The listing builds one solid part. Answer for the finished solid, in the listing's coordinates (mm). A direction names the side the tool comes from. Coordinates: 2 decimals unless noted, no trailing zeros. Order: outer loops, then holes, each group sorted by start corner. A loop starts at its lowest first (then second) coordinate and runs counter-clockwise, first axis right, second up. Notation, with made-up numbers: (16, -22) -> (66, -22) arc R24 cw to (66, -1) -> close; hole circle Ø2 at (-39, 12). An arc over 180 degrees is marked (long way). Answer in a Markdown table with one row per item.
```python
from build123d import *

# Parameters (mm, degrees)
CUT_EXTRUDE2_DEPTH      = 28.696934518
CUT_EXTRUDE2_DEPTH_BACK = 28.696934518
SKETCH10_R              = 0.75


with BuildPart() as part:
    # Sketch1 → Revolve1 (revolve)
    with BuildSketch(Plane(origin=(0, 0, 0), x_dir=(0, 0, -1), z_dir=(1, 0, 0))):
        Polygon((-6.059175667, 3.611199877), (-6.059175667, -4.388800123), (-4.559175656, -4.388756431), (-4.559175656, -2.888756431), (-3.059175668, -2.88856746), (-3.059175668, -4.388756431), (-1.059175668, -4.388756431), (-0.059175667, -1.888800123), (-0.059175667, 0.111199877), (-0.809175667, 0.611199877), (-0.809175667, 3.611199877), align=None)
    revolve(axis=Axis((0, 4.111199877, -8.940824333), (0, -1, 0)))

    # Sketch10 → Cut-Extrude2 (cut, two sides: drawn at the far end of the back side and taken through both)
    with BuildSketch(Plane(origin=(0, 5.926037439, -14.814834675), x_dir=(1, 0, 0), z_dir=(0, -0.37139627193644054, 0.9284744526327656)).offset(-CUT_EXTRUDE2_DEPTH_BACK)):
        with Locations(Location((4.041684761, -9.017, 0), (0, 0, 270))):
            Circle(SKETCH10_R)
    extrude(amount=CUT_EXTRUDE2_DEPTH + CUT_EXTRUDE2_DEPTH_BACK, mode=Mode.SUBTRACT)


solid = part.part
```
(1) A cutting plane is placed at A-A, the plane x = 0. Determine the outline of the cut face in (y, z), then the cut area to 3 significant figures.
Check values:
| item | result |
|---|---|
| outline | (-4.39, -23.94) -> (3.61, -23.94) -> (3.61, -18.69) -> (0.61, -18.69) -> (0.11, -17.94) -> (-1.89, -17.94) -> (-4.39, -18.94) -> (-4.39, -20.94) -> (-2.89, -20.94) -> (-2.89, -22.44) -> (-4.39, -22.44) -> close; (-4.39, 1.06) -> (-1.89, 0.06) -> (0.11, 0.06) -> (0.61, 0.81) -> (3.61, 0.81) -> (3.61, 6.06) -> (-4.39, 6.06) -> (-4.39, 4.56) -> (-2.89, 4.56) -> (-2.89, 3.06) -> (-4.39, 3.06) -> close |
| area | 84.1 mm² |
(2) Flat-ended cylindrical pins translate along their axes: pin 1 (15.5 mm diameter, centred on x = 0, z = -8.94, fed in from +Y) (3 decimals); pin 2 (1 mm diameter, centred on x = 3, z = 0.5, fed in from -Y); pin 3 (1 mm diameter, centred on y = 0, z = -15, fed in from +X). Find the tip coordinate at first contact, or state that the pin passes through.
Check values:
| item | result |
|---|---|
| pin 1 | through |
| pin 2 | y = -4.39 |
| pin 3 | x = 13.93 |
(3) For a pull along X with two mould halves and no side action, classify faces 1 (the cylindrical face through (-0.4, -0.87, -17.93)), 2 (the cylindrical face through (-6.59, 2.132, -16.127)), 3 (the cylindrical face through (-4.506, -0.445, 5.367)), 4 (the flat face through (10, 3.611, -9)) as released by +X, released by -X, zero draft, split by the parting line, or undercut.
Check values:
| item | result |
|---|---|
| face 1 | undercut |
| face 2 | undercut |
| face 3 | split by the parting line |
| face 4 | zero draft |
(4) Find the intervals of material crossed by line 1 along X through (y, z) = (-3.5, -20); line 2 along Z through (x, y) = (-8.5, 2.25); line 3 along X through (y, z) = (-1.5, -1.5), in increasing order. Write a range as from..to.
Check values:
| item | result |
|---|---|
| line 1 | -10.13..-7.74, -4.66..4.66, 7.74..10.13 |
| line 2 | -21.3..-13.72, -4.16..3.42 |
| line 3 | -13.02..-5.06, 5.06..13.02 |
(5) Which of the six approach directions +Z, -Z, +X, -X, +Y, -Y give full straight-line access (tool end or side, diameter ignored) to faces 5 (the cylindrical face through (4.075, -0.846, -20.147)), 6 (the cylindrical face through (-0.594, -3.628, -22.428))?
Check values:
| item | result |
|---|---|
| face 5 | none |
| face 6 | -Y |
(6) A cutting plane is placed at B-B, the plane y = 2.5. Determine the outline of the cut face in (x, z).
Check values:
| item | result |
|---|---|
| outline | circle Ø30 at (0, -8.94); hole circle Ø19.5 at (0, -8.94) |
